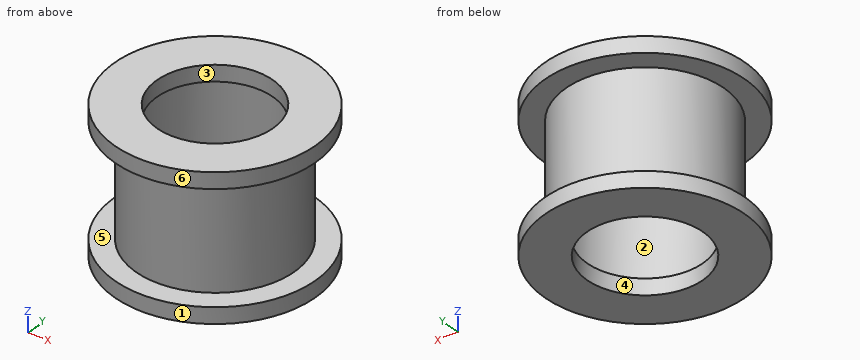
from build123d import *

# Parameters (mm, degrees)
ESQUISSE1_R        = 9.5
ESQUISSE1_R_2      = 6.45
ESQUISSE1_R_3      = 5.5
BOSS_EXTRU_1_DEPTH = 1.5
ESQUISSE1_3_R      = 6.45
ESQUISSE1_3_R_2    = 5.5
BOSS_EXTRU_4_DEPTH = 1.5
ESQUISSE6_R        = 7.5
ESQUISSE6_R_2      = 6.5
BOSS_EXTRU_5_DEPTH = 10.5
ESQUISSE7_R        = 9.5
ESQUISSE7_R_2      = 7.5
ESQUISSE7_R_3      = 6.5
ESQUISSE7_R_4      = 5.5
BOSS_EXTRU_6_DEPTH = 1.5


with BuildPart() as part:
    # Esquisse1 → Boss.-Extru.1 (new body)
    # profile 1 of 2: a face of its own
    with BuildSketch(Plane.XY):
        Circle(ESQUISSE1_R)
        Circle(ESQUISSE1_R_2, mode=Mode.SUBTRACT)
    # profile 2 of 2: a face of its own
    with BuildSketch(Plane.XY):
        Circle(ESQUISSE1_R_2)
        Circle(ESQUISSE1_R_3, mode=Mode.SUBTRACT)
    extrude(amount=BOSS_EXTRU_1_DEPTH)

    # Esquisse1<3> → Boss.-Extru.4 (add)
    with BuildSketch(Plane.XY):
        Circle(ESQUISSE1_3_R)
        Circle(ESQUISSE1_3_R_2, mode=Mode.SUBTRACT)
    extrude(amount=BOSS_EXTRU_4_DEPTH)

    # Esquisse6 → Boss.-Extru.5 (add)
    with BuildSketch(Plane.XY.offset(1.5)):
        with Locations(Location((0, 0, 0), (0, 0, 180))):
            Circle(ESQUISSE6_R)
        with Locations(Location((0, 0, 0), (0, 0, 180))):
            Circle(ESQUISSE6_R_2, mode=Mode.SUBTRACT)
    extrude(amount=BOSS_EXTRU_5_DEPTH)

    # Esquisse7 → Boss.-Extru.6 (add)
    # profile 1 of 3: a face of its own
    with BuildSketch(Plane.XY.offset(12)):
        Circle(ESQUISSE7_R)
        with Locations(Location((0, 0, 0), (0, 0, 180))):
            Circle(ESQUISSE7_R_2, mode=Mode.SUBTRACT)
    # profile 2 of 3: a face of its own
    with BuildSketch(Plane.XY.offset(12)):
        with Locations(Location((0, 0, 0), (0, 0, 180))):
            Circle(ESQUISSE7_R_2)
        with Locations(Location((0, 0, 0), (0, 0, 180))):
            Circle(ESQUISSE7_R_3, mode=Mode.SUBTRACT)
    # profile 3 of 3: a face of its own
    with BuildSketch(Plane.XY.offset(12)):
        with Locations(Location((0, 0, 0), (0, 0, 180))):
            Circle(ESQUISSE7_R_3)
        Circle(ESQUISSE7_R_4, mode=Mode.SUBTRACT)
    extrude(amount=BOSS_EXTRU_6_DEPTH)


solid = part.part
Geometry check sheet. Reference: the model listing, model coordinates, mm. Face numbers are marked on the shaded views. A direction names the side the tool comes from. Give positions to 0.01 mm unless a question says otherwise; leave off trailing zeros. Write each loop counter-clockwise with the first axis right and the second up, starting at its lowest first coordinate (ties: lowest second). Pieces come first, ordered by that corner, then holes.
1) Cross-section at C-C (z = 4.75). Record the boundary of the cut face in (x, y), plus the area to 3 significant figures.
Values follow:
outline: circle Ø15 at (0, 0); hole circle Ø13 at (0, 0)
area: 44.0 mm2
2) Thickness scan on line 1 (Z direction, x = -2.75, y = 8.75); line 2 (Y direction, x = 0, z = 12.8); line 3 (Y direction, x = -1, z = 1.75). Record the ranges inside material, lowest first.
Values follow:
line 1: z = 0 to 1.5, 12 to 13.5
line 2: y = -9.5 to -5.5, 5.5 to 9.5
line 3: y = -7.43 to -6.42, 6.42 to 7.43
3) Cross-section at D-D (y = -6.25). Record the boundary of the cut face in (x, z), plus the area to 3 significant figures.
Values follow:
outline: (-7.15, 0) - (7.15, 0) - (7.15, 1.5) - (4.15, 1.5) - (4.15, 12) - (7.15, 12) - (7.15, 13.5) - (-7.15, 13.5) - (-7.15, 12) - (-4.15, 12) - (-4.15, 1.5) - (-7.15, 1.5) - close; hole (-1.79, 1.5) - (1.79, 1.5) - (1.79, 12) - (-1.79, 12) - close
area: 92.5 mm2
4) Go/stop test with flat-tipped pins: pin 1 Ø5 at (y, z) = (-3, 3) entering from -X; pin 2 Ø2 at (x, z) = (-1, 7) entering from -Y; pin 3 Ø8 at (y, z) = (1, 3.5) entering from +X; pin 4 Ø8 at (y, z) = (-1.5, 7) entering from -X. Record where each tip stops, or that it passes through.
Values follow:
pin 1: stops at x = -9.45
pin 2: stops at y = -7.5
pin 3: stops at x = 9.5
pin 4: stops at x = -7.5
5) Release check for a two-part mould opening along Y. For the marked faces 3, 4, 5 and 6 record: released by +Y, released by -Y, zero draft, split by the parting line, or undercut.
Values follow:
face 3: undercut
face 4: undercut
face 5: zero draft
face 6: split by the parting line
6) Set-up check for the marked faces 1 and 2: record each of +Z, -Z, +X, -X, +Y, -Y from which the full face is reachable in a straight line by a thin tool's end or side.
Values follow:
face 1: +Z, -Z
face 2: none
7) Cross-section at A-A (x = 0). Record the boundary of the cut face in (y, z), plus the area to 3 significant figures.
Values follow:
outline: (-9.5, 0) - (-5.5, 0) - (-5.5, 1.5) - (-6.5, 1.5) - (-6.5, 12) - (-5.5, 12) - (-5.5, 13.5) - (-9.5, 13.5) - (-9.5, 12) - (-7.5, 12) - (-7.5, 1.5) - (-9.5, 1.5) - close; (5.5, 0) - (9.5, 0) - (9.5, 1.5) - (7.5, 1.5) - (7.5, 12) - (9.5, 12) - (9.5, 13.5) - (5.5, 13.5) - (5.5, 12) - (6.5, 12) - (6.5, 1.5) - (5.5, 1.5) - close
area: 45.0 mm2
